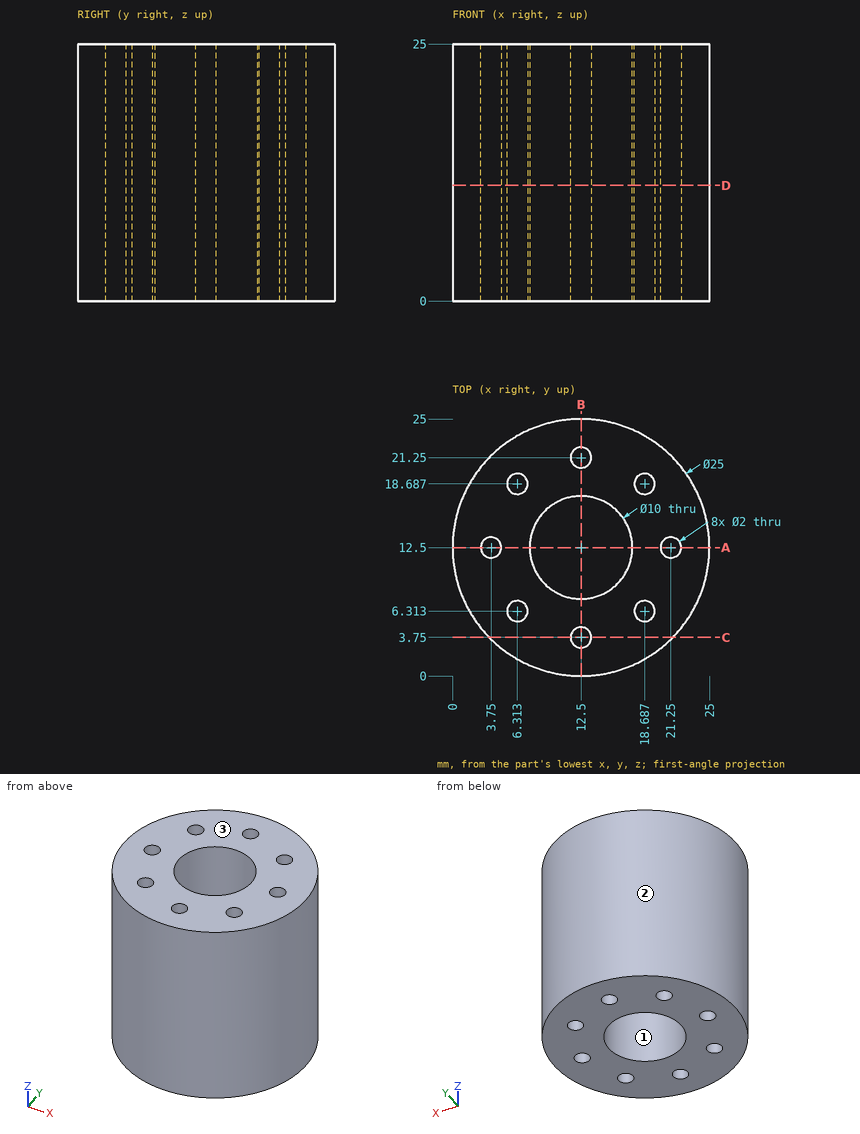
Print and shaded views of the part. All mm, measured from the part's lowest x, y and z. Give positions to 0.01 mm unless a question says otherwise; leave off trailing zeros. Write each loop counter-clockwise with the first axis right and the second up, starting at its lowest first coordinate (ties: lowest second). Pieces come first, ordered by that corner, then holes. Notation, with made-up numbers: M 62.5,-33 L 87.5,-33 A20 ccw 87.5,1 Z; hole C 25,-10.5 d2. An arc over 180 degrees is marked long. Use a Markdown table: item, result.
1) Cut at A-A (y = 12.5). List the corners of the cut face in (x, z), and give its area (3 significant figures).
Responses:
| item | result |
|---|---|
| outline | M 0,0 L 2.75,0 L 2.75,25 L 0,25 Z; M 4.75,0 L 7.5,0 L 7.5,25 L 4.75,25 Z; M 17.5,0 L 20.25,0 L 20.25,25 L 17.5,25 Z; M 22.25,0 L 25,0 L 25,25 L 22.25,25 Z |
| area | 275 mm2 |
2) Cut at C-C (y = 3.75). List the corners of the cut face in (x, z).
Responses:
| item | result |
|---|---|
| outline | M 3.57,0 L 11.5,0 L 11.5,25 L 3.57,25 Z; M 13.5,0 L 21.43,0 L 21.43,25 L 13.5,25 Z |
3) Cut at D-D (z = 11.25). Give the number of separate pieces and of enclosed holes in the cut face, and give its area (3 significant figures).
Responses:
| item | result |
|---|---|
| separate pieces | 1 |
| enclosed holes | 9 |
| area | 387 mm2 |
4) Pull direction Y, two halves, no side cores. Call the marked faces 1, 2 and 3: +Y half, -Y half, draft (parallel to the pull), parting line (faces both ways), or undercut.
Responses:
| item | result |
|---|---|
| face 1 | undercut |
| face 2 | parting line |
| face 3 | draft |
5) Pin check, flat tips, straight feed: pin 1 (1.8 mm diameter, centred on x = 6.31, y = 6.31, fed in from +Z); pin 2 (1 mm diameter, centred on y = 15, z = 4.5, fed in from -X); pin 3 (8 mm diameter, centred on x = 3.5, z = 13.5, fed in from +Y); pin 4 (1.5 mm diameter, centred on y = 7.5, z = 12.5, fed in from +X) (1 decimal). Stop position of each tip, or through.
Responses:
| item | result |
|---|---|
| pin 1 | passes through |
| pin 2 | stops at x = 0.16 |
| pin 3 | stops at y = 23.96 |
| pin 4 | stops at x = 24.3 |
6) Drill centre lines: line 1 (Y direction, x = 12.5, z = 12.25); line 2 (Y direction, x = 19.5, z = 4.75) (1 decimal); line 3 (X direction, y = 7, z = 9.25) (1 decimal). Where is each one in solid material? Low to high. Write a range as from..to.
Responses:
| item | result |
|---|---|
| line 1 | y = 0..2.75, 4.75..7.5, 17.5..20.25, 22.25..25 |
| line 2 | y = 2.1..5.7, 6.9..18.1, 19.3..22.9 |
| line 3 | x = 1.3..5.6, 7..18, 19.4..23.7 |
